Job drawing, mm, ordinate dimensions from the low corner. One solid piece. A direction names the side the tool comes from. Give positions to 0.01 mm unless a question says otherwise; leave off trailing zeros. Order: outer loops, then holes, each group sorted by start corner. A loop starts at its lowest first (then second) coordinate and runs counter-clockwise, first axis right, second up. Notation, with made-up numbers: M 6,32.25 L 53,32.25 A23 ccw 53,47.25 Z; hole C -25.75,42.5 d8. An arc over 180 degrees is marked long. One line per question, with ' | ' between items.
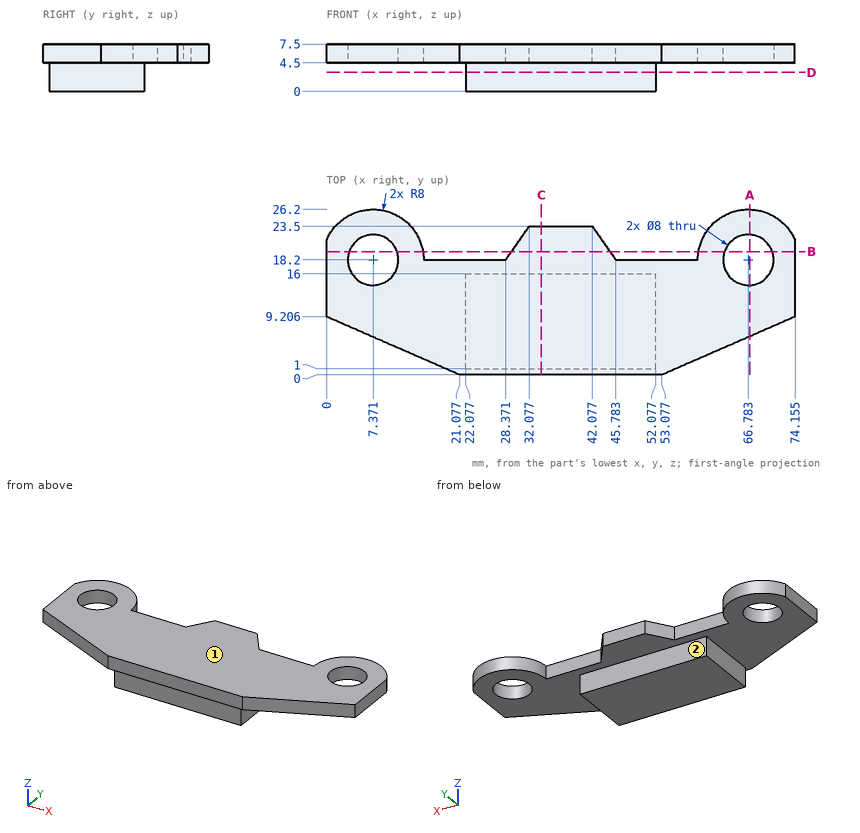
1. Slice it at D-D on z = 3. Give the cut face in (x, y), then the cut area to 3 significant figures.
Worked out:
outline: M 22.08,1 L 52.08,1 L 52.08,16 L 22.08,16 Z | area: 450 mm2
2. Slice it at B-B on y = 19.5. Give the cut face in (x, z) (1 decimal).
Worked out:
outline: M 0,4.5 L 3.6,4.5 L 3.6,7.5 L 0,7.5 Z; M 11.2,4.5 L 15.3,4.5 L 15.3,7.5 L 11.2,7.5 Z; M 29.3,4.5 L 44.9,4.5 L 44.9,7.5 L 29.3,7.5 Z; M 58.9,4.5 L 63,4.5 L 63,7.5 L 58.9,7.5 Z; M 70.6,4.5 L 74.2,4.5 L 74.2,7.5 L 70.6,7.5 Z
3. Slice it at C-C on x = 34. Give the cut face in (y, z).
Worked out:
outline: M 0,4.5 L 1,4.5 L 1,0 L 16,0 L 16,4.5 L 23.5,4.5 L 23.5,7.5 L 0,7.5 Z
4. Tool access for the marked faces 1 and 2: list every direction of +Z, -Z, +X, -X, +Y, -Y with a clear straight run to the whole face (end or side of a thin tool).
Worked out:
face 1: +Z, +X, -X, +Y, -Y | face 2: -Z, +X, -X, +Y
5. Probe L1, parallel to X at y = 17, z = 6.5 (1 decimal); L2, parallel to X at y = 20, z = 5 (1 decimal); L3, parallel to Z at x = 52, y = 18. List the from-to ranges inside material, lowest first. Write a range as from..to.
Worked out:
L1: x = 0..3.6, 11.2..63, 70.6..74.2 | L2: x = 0..3.8, 10.9..15.2, 29.6..44.5, 59..63.2, 70.4..74.2 | L3: z = 4.5..7.5
6. Slice it at A-A on x = 67. Give the cut face in (y, z), then the cut area to 3 significant figures.
Worked out:
outline: M 6.08,4.5 L 14.21,4.5 L 14.21,7.5 L 6.08,7.5 Z; M 22.19,4.5 L 26.2,4.5 L 26.2,7.5 L 22.19,7.5 Z | area: 36.4 mm2
7. Drop flat-ended pins along their axis: pin 1 (2 mm diameter, centred on x = 31, z = 2.5, fed in from -Y); pin 2 (6.5 mm diameter, centred on x = 66.78, y = 18.2, fed in from +Z); pin 3 (5 mm diameter, centred on x = 40, y = 20.5, fed in from -Z); pin 4 (3 mm diameter, centred on x = 30.5, z = 6.5, fed in from +Y). Give the stop position or say it passes through.
Worked out:
pin 1: stops at y = 1 | pin 2: passes through | pin 3: stops at z = 4.5 | pin 4: stops at y = 23.39
